```python
from build123d import *

# Parameters (mm, degrees)
F0_R     = 12.7
F0_R_2   = 6.35
F1_DEPTH = 10
F2_DEPTH = 20
F3_W     = 3
F3_H     = 1
F4_DEPTH = 7


with BuildPart() as f1:
    # F0 (on Top) → F1 (new body)
    with BuildSketch(Plane.XY):
        Circle(F0_R)
        Circle(F0_R_2, mode=Mode.SUBTRACT)
    extrude(amount=F1_DEPTH)

    # F0 (on Top) → F2 (join)
    with BuildSketch(Plane.XY):
        Circle(F0_R_2)
    extrude(amount=F2_DEPTH)

    # F3 (on face) → F4 (join)
    with BuildSketch(Plane.XY.offset(20)):
        Rectangle(F3_W, F3_H)
    extrude(amount=F4_DEPTH)


solid = f1.part
```
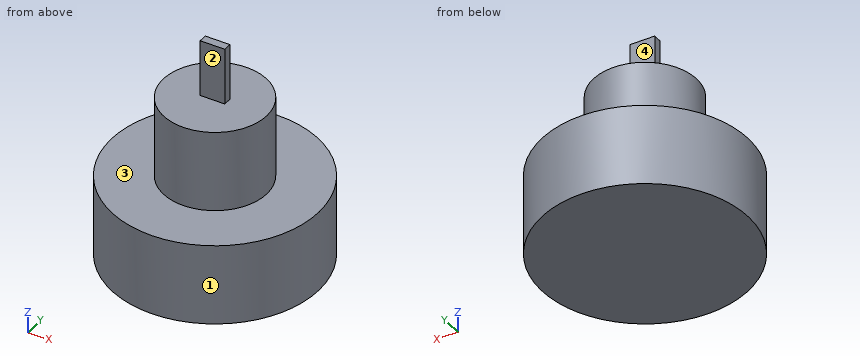
Source: CAD feature listing. Evaluate the final solid. Frame: model axes, mm. Face numbers are marked on the shaded views. A direction names the side the tool comes from. Give positions to 0.01 mm unless a question says otherwise; leave off trailing zeros. Loops run counter-clockwise (first coordinate to the right, second up) from the corner with the lowest first, then second, coordinate; pieces in that order, holes last. Notation, with made-up numbers: (14.5, 79) - (33.5, 79) arc R12 cw to (33.5, 90) - close; hole circle Ø11 at (-40, 77). An arc over 180 degrees is marked (long way). Use CSV: the item, a comma, the result in double quotes. Start each with the question number.
1. Reachability of the marked faces 1, 2, 3 and 4 from +Z, -Z, +X, -X, +Y, -Y: full face, straight path, thin tool, end or side. Return the list, or none.
2. Ray query, L1, parallel to Z at x = -10.75, y = -2.5; L2, parallel to Y at x = -1, z = 23; L3, parallel to Z at x = -2.75, y = 3.25. Return the intervals inside material, ascending.
3. Section D-D (y = 5.5). Output: boundary loops of the cut face in (x, z).
4. Section B-B (y = 0). Output: boundary loops of the cut face in (x, z).
5. Pin query (flat end, axial travel): pin 1 (1.5 mm diameter, centred on y = 1, z = 8.5, fed in from -X); pin 2 (0.9 mm diameter, centred on x = 0, z = 22.5, fed in from -Y); pin 3 (1 mm diameter, centred on x = 2.5, z = 5, fed in from -Y). Return the tip coordinate at first contact, or that it passes through.
6. Section C-C (z = 21). Output: boundary loops of the cut face in (x, y).
7. Section A-A (x = 0). Output: boundary loops of the cut face in (y, z).
Response:
1,face 1,"+Z, -Z"
1,face 2,"+Z, +X, -X, -Y"
1,face 3,"+Z"
1,face 4,"+Z, +X, -X, +Y"
2,L1,"0 to 10"
2,L2,"-0.5 to 0.5"
2,L3,"0 to 20"
3,outline,"(-11.45, 0) - (11.45, 0) - (11.45, 10) - (3.17, 10) - (3.17, 20) - (-3.17, 20) - (-3.17, 10) - (-11.45, 10) - close"
4,outline,"(-12.7, 0) - (12.7, 0) - (12.7, 10) - (6.35, 10) - (6.35, 20) - (1.5, 20) - (1.5, 27) - (-1.5, 27) - (-1.5, 20) - (-6.35, 20) - (-6.35, 10) - (-12.7, 10) - close"
5,pin 1,"x = -12.7"
5,pin 2,"y = -0.5"
5,pin 3,"y = -12.54"
6,outline,"(-1.5, -0.5) - (1.5, -0.5) - (1.5, 0.5) - (-1.5, 0.5) - close"
7,outline,"(-12.7, 0) - (12.7, 0) - (12.7, 10) - (6.35, 10) - (6.35, 20) - (0.5, 20) - (0.5, 27) - (-0.5, 27) - (-0.5, 20) - (-6.35, 20) - (-6.35, 10) - (-12.7, 10) - close"
